from build123d import *

# Parameters (mm, degrees)
BOSS_EXTRUDE1_DEPTH = 5
CUT_EXTRUDE1_REACH  = 58.403
SKETCH2_R           = 1.75
SKETCH4_W           = 75
SKETCH4_H           = 60
BOSS_EXTRUDE2_DEPTH = 5
CUT_EXTRUDE2_REACH  = 90.459
SKETCH3_R           = 2.5
SKETCH3_W           = 23
SKETCH3_H           = 42
FILLET1_R           = 25
FILLET2_R           = 5
FILLET3_R           = 2
FILLET4_R           = 1
BOSS_EXTRUDE3_DEPTH = 10
LPATTERN1_COUNT     = 2
LPATTERN1_PITCH     = 50
CUT_EXTRUDE3_REACH  = 95.708
SKETCH7_R           = 5


with BuildPart() as part:
    # Sketch1 → Boss-Extrude1 (new body)
    with BuildSketch(Plane(origin=(0, 0, 0), x_dir=(0, 0, -1), z_dir=(1, 0, 0))):
        with BuildLine():
            ThreePointArc((-30, -17.5), (0, -47.5), (30, -17.5))
            Line((30, -17.5), (30, 17.5))
            Line((30, 17.5), (-30, 17.5))
            Line((-30, 17.5), (-30, -17.5))
        make_face()
    extrude(amount=BOSS_EXTRUDE1_DEPTH)

    # Sketch2 → Cut-Extrude1 (cut, up to next)
    with BuildSketch(Plane(origin=(5, 0, 0), x_dir=(0, 0, -1), z_dir=(1, 0, 0)), mode=Mode.PRIVATE) as cut_extrude1_sk1:
        with Locations((-15, -32.5)):
            Circle(SKETCH2_R)
    cut_extrude1_tool1 = extrude(cut_extrude1_sk1.sketch, amount=-CUT_EXTRUDE1_REACH, mode=Mode.PRIVATE) & part.part
    # Sketch2 → Cut-Extrude1 (cut, up to next)
    with BuildSketch(Plane(origin=(5, 0, 0), x_dir=(0, 0, -1), z_dir=(1, 0, 0)), mode=Mode.PRIVATE) as cut_extrude1_sk2:
        with Locations((15, -32.5)):
            Circle(SKETCH2_R)
    cut_extrude1_tool2 = extrude(cut_extrude1_sk2.sketch, amount=-CUT_EXTRUDE1_REACH, mode=Mode.PRIVATE) & part.part
    # Sketch2 → Cut-Extrude1 (cut, up to next)
    with BuildSketch(Plane(origin=(5, 0, 0), x_dir=(0, 0, -1), z_dir=(1, 0, 0)), mode=Mode.PRIVATE) as cut_extrude1_sk3:
        with Locations((-15, -2.5)):
            Circle(SKETCH2_R)
    cut_extrude1_tool3 = extrude(cut_extrude1_sk3.sketch, amount=-CUT_EXTRUDE1_REACH, mode=Mode.PRIVATE) & part.part
    # Sketch2 → Cut-Extrude1 (cut, up to next)
    with BuildSketch(Plane(origin=(5, 0, 0), x_dir=(0, 0, -1), z_dir=(1, 0, 0)), mode=Mode.PRIVATE) as cut_extrude1_sk4:
        with Locations((0, -2.5)):
            Circle(SKETCH2_R)
    cut_extrude1_tool4 = extrude(cut_extrude1_sk4.sketch, amount=-CUT_EXTRUDE1_REACH, mode=Mode.PRIVATE) & part.part
    # Sketch2 → Cut-Extrude1 (cut, up to next)
    with BuildSketch(Plane(origin=(5, 0, 0), x_dir=(0, 0, -1), z_dir=(1, 0, 0)), mode=Mode.PRIVATE) as cut_extrude1_sk5:
        with Locations((15, -2.5)):
            Circle(SKETCH2_R)
    cut_extrude1_tool5 = extrude(cut_extrude1_sk5.sketch, amount=-CUT_EXTRUDE1_REACH, mode=Mode.PRIVATE) & part.part
    # Sketch2 → Cut-Extrude1 (cut, up to next)
    with BuildSketch(Plane(origin=(5, 0, 0), x_dir=(0, 0, -1), z_dir=(1, 0, 0)), mode=Mode.PRIVATE) as cut_extrude1_sk6:
        with Locations((0, -32.5)):
            Circle(SKETCH2_R)
    cut_extrude1_tool6 = extrude(cut_extrude1_sk6.sketch, amount=-CUT_EXTRUDE1_REACH, mode=Mode.PRIVATE) & part.part
    # Sketch2 → Cut-Extrude1 (cut, up to next)
    with BuildSketch(Plane(origin=(5, 0, 0), x_dir=(0, 0, -1), z_dir=(1, 0, 0)), mode=Mode.PRIVATE) as cut_extrude1_sk7:
        with Locations((-15, -17.5)):
            Circle(SKETCH2_R)
    cut_extrude1_tool7 = extrude(cut_extrude1_sk7.sketch, amount=-CUT_EXTRUDE1_REACH, mode=Mode.PRIVATE) & part.part
    # Sketch2 → Cut-Extrude1 (cut, up to next)
    with BuildSketch(Plane(origin=(5, 0, 0), x_dir=(0, 0, -1), z_dir=(1, 0, 0)), mode=Mode.PRIVATE) as cut_extrude1_sk8:
        with Locations((15, -17.5)):
            Circle(SKETCH2_R)
    cut_extrude1_tool8 = extrude(cut_extrude1_sk8.sketch, amount=-CUT_EXTRUDE1_REACH, mode=Mode.PRIVATE) & part.part
    add(cut_extrude1_tool1.solids().sort_by_distance((5, -32.5, 15))[0], mode=Mode.SUBTRACT)
    add(cut_extrude1_tool2.solids().sort_by_distance((5, -32.5, -15))[0], mode=Mode.SUBTRACT)
    add(cut_extrude1_tool3.solids().sort_by_distance((5, -2.5, 15))[0], mode=Mode.SUBTRACT)
    add(cut_extrude1_tool4.solids().sort_by_distance((5, -2.5, 0))[0], mode=Mode.SUBTRACT)
    add(cut_extrude1_tool5.solids().sort_by_distance((5, -2.5, -15))[0], mode=Mode.SUBTRACT)
    add(cut_extrude1_tool6.solids().sort_by_distance((5, -32.5, 0))[0], mode=Mode.SUBTRACT)
    add(cut_extrude1_tool7.solids().sort_by_distance((5, -17.5, 15))[0], mode=Mode.SUBTRACT)
    add(cut_extrude1_tool8.solids().sort_by_distance((5, -17.5, -15))[0], mode=Mode.SUBTRACT)

    # Sketch4 → Boss-Extrude2 (add)
    with BuildSketch(Plane(origin=(0, 17.5, 0), x_dir=(1, 0, 0), z_dir=(0, 1, 0))):
        with Locations((37.5, 0)):
            Rectangle(SKETCH4_W, SKETCH4_H)
    extrude(amount=BOSS_EXTRUDE2_DEPTH)

    # Sketch3 → Cut-Extrude2 (cut, up to next)
    with BuildSketch(Plane(origin=(30, 22.5, 0), x_dir=(0, 0, -1), z_dir=(0, 1, 0)), mode=Mode.PRIVATE) as cut_extrude2_sk1:
        with Locations(Location((-5.25, 17.65, 0), (0, 0, 180))):
            Circle(SKETCH3_R)
    cut_extrude2_tool1 = extrude(cut_extrude2_sk1.sketch, amount=-CUT_EXTRUDE2_REACH, mode=Mode.PRIVATE) & part.part
    # Sketch3 → Cut-Extrude2 (cut, up to next)
    with BuildSketch(Plane(origin=(30, 22.5, 0), x_dir=(0, 0, -1), z_dir=(0, 1, 0)), mode=Mode.PRIVATE) as cut_extrude2_sk2:
        with Locations(Location((5.25, 17.65, 0), (0, 0, 180))):
            Circle(SKETCH3_R)
    cut_extrude2_tool2 = extrude(cut_extrude2_sk2.sketch, amount=-CUT_EXTRUDE2_REACH, mode=Mode.PRIVATE) & part.part
    # Sketch3 → Cut-Extrude2 (cut, up to next)
    with BuildSketch(Plane(origin=(30, 22.5, 0), x_dir=(0, 0, -1), z_dir=(0, 1, 0)), mode=Mode.PRIVATE) as cut_extrude2_sk3:
        with Locations(Location((5.25, -32.65, 0), (0, 0, 180))):
            Circle(SKETCH3_R)
    cut_extrude2_tool3 = extrude(cut_extrude2_sk3.sketch, amount=-CUT_EXTRUDE2_REACH, mode=Mode.PRIVATE) & part.part
    # Sketch3 → Cut-Extrude2 (cut, up to next)
    with BuildSketch(Plane(origin=(30, 22.5, 0), x_dir=(0, 0, -1), z_dir=(0, 1, 0)), mode=Mode.PRIVATE) as cut_extrude2_sk4:
        with Locations(Location((-5.25, -32.65, 0), (0, 0, 180))):
            Circle(SKETCH3_R)
    cut_extrude2_tool4 = extrude(cut_extrude2_sk4.sketch, amount=-CUT_EXTRUDE2_REACH, mode=Mode.PRIVATE) & part.part
    # Sketch3 → Cut-Extrude2 (cut, up to next)
    with BuildSketch(Plane(origin=(30, 22.5, 0), x_dir=(0, 0, -1), z_dir=(0, 1, 0)), mode=Mode.PRIVATE) as cut_extrude2_sk5:
        with Locations((0, -7.5)):
            Rectangle(SKETCH3_W, SKETCH3_H)
    cut_extrude2_tool5 = extrude(cut_extrude2_sk5.sketch, amount=-CUT_EXTRUDE2_REACH, mode=Mode.PRIVATE) & part.part
    add(cut_extrude2_tool1.solids().sort_by_distance((12.35, 22.5, 5.25))[0], mode=Mode.SUBTRACT)
    add(cut_extrude2_tool2.solids().sort_by_distance((12.35, 22.5, -5.25))[0], mode=Mode.SUBTRACT)
    add(cut_extrude2_tool3.solids().sort_by_distance((62.65, 22.5, -5.25))[0], mode=Mode.SUBTRACT)
    add(cut_extrude2_tool4.solids().sort_by_distance((62.65, 22.5, 5.25))[0], mode=Mode.SUBTRACT)
    add(cut_extrude2_tool5.solids().sort_by_distance((37.5, 22.5, 0))[0], mode=Mode.SUBTRACT)

    # Fillet1
    fillet1_edges = [part.edges().sort_by_distance(p)[0] for p in [
        (75, 20, 30),
        (75, 20, -30),
    ]]
    fillet(fillet1_edges, radius=FILLET1_R)

    # Fillet2
    fillet2_edges = [part.edges().sort_by_distance(p)[0] for p in [
        (0, 22.5, 0),
    ]]
    fillet(fillet2_edges, radius=FILLET2_R)

    # Fillet3
    fillet3_edges = [part.edges().sort_by_distance(p)[0] for p in [
        (5, 17.5, 0),
    ]]
    fillet(fillet3_edges, radius=FILLET3_R)

    # Fillet4
    fillet4_edges = [part.edges().sort_by_distance(p)[0] for p in [
        (58.5, 20, -11.5),
        (58.5, 20, 11.5),
        (16.5, 20, 11.5),
        (16.5, 20, -11.5),
    ]]
    fillet(fillet4_edges, radius=FILLET4_R)

    # Sketch6 → Boss-Extrude3 (add)
    with BuildSketch(Plane.XY.offset(30)):
        Polygon((18.5, 17.5), (5, 2.743645437), (5, 17.5), align=None)
    boss_extrude3 = extrude(amount=-BOSS_EXTRUDE3_DEPTH)

    # LPattern1: Boss-Extrude3 ×2
    with Locations(*[(0, 0, -i * LPATTERN1_PITCH) for i in range(1, LPATTERN1_COUNT)]):
        add(boss_extrude3)

    # Sketch7 → Cut-Extrude3 (cut, up to next)
    with BuildSketch(Plane.ZY, mode=Mode.PRIVATE) as cut_extrude3_sk1:
        with Locations((0, -17.5)):
            Circle(SKETCH7_R)
    cut_extrude3_tool1 = extrude(cut_extrude3_sk1.sketch, amount=-CUT_EXTRUDE3_REACH, mode=Mode.PRIVATE) & part.part
    add(cut_extrude3_tool1.solids().sort_by_distance((0, -17.5, 0))[0], mode=Mode.SUBTRACT)


solid = part.part
Part model, mm, in its own coordinate system. A direction names the side the tool comes from. Coordinates: 2 decimals unless noted, no trailing zeros. Loops run counter-clockwise (first coordinate to the right, second up) from the corner with the lowest first, then second, coordinate; pieces in that order, holes last. Notation, with made-up numbers: (-22.5, 84) - (32.5, 84) arc R24 ccw to (32.5, 113) - close; hole circle Ø5 at (49.25, 16). An arc over 180 degrees is marked (long way). Write each question's results on one line, items separated by ' | '. Start each with the question number.
Q1. Drop flat-ended pins along their axis: pin 1 Ø2 at (y, z) = (-17.5, 15) entering from -X; pin 2 Ø8 at (x, z) = (23.5, -24) entering from -Y; pin 3 Ø6 at (y, z) = (-8.5, -13) entering from +X. Give the stop position or say it passes through.
Q2. Slice it at A-A on x = 34.5. Give the cut face in (y, z).
Q3. Slice it at B-B on z = 0. Give the cut face in (x, y).
Q4. Probe line 1 along Z through (x, y) = (2, -32); line 2 along X through (y, z) = (19.1, 5.25); line 3 along Y through (x, z) = (2, -15). List the from-to ranges inside material, lowest first.
Q5. Slice it at D-D on z = -15. Give the cut face in (x, y), and give its area (3 significant figures).
Q6. Slice it at C-C on y = -32.5. Give the cut face in (x, z), and give its area (3 significant figures).
Q7. Which spindle directions (+Z, -Z, +X, -X, +Y, -Y) get a long thin tool onto all of the face, cutting with end or side? Do faces 4 (the flat face through (38, 20, -11.5)), 5 (the cylindrical face through (2.54, -4.21, 0.38)), 6 (the flat face through (41, 17.5, 13)). Say none if no direction does.
Q8. Two-plate mould, pull along Z, no slides. Class faces 1 (the flat face through (14, 13, 30)), 2 (the cylindrical face through (60.21, 20.04, -5.79)), 3 (the cylindrical face through (1.5, 21.07, -0.42)): +Z half, -Z half, draft (parallel to the pull), parting line (faces both ways), or undercut.
Answer:
1) pin 1: passes through | pin 2: stops at y = 17.5 | pin 3: stops at x = 5
2) outline: (17.5, -30) - (22.5, -30) - (22.5, -11.5) - (17.5, -11.5) - close; (17.5, 11.5) - (22.5, 11.5) - (22.5, 30) - (17.5, 30) - close
3) outline: (0, -47.5) - (5, -47.5) - (5, -34.25) - (0, -34.25) - close; (0, -30.75) - (5, -30.75) - (5, -22.5) - (0, -22.5) - close; (0, -12.5) - (5, -12.5) - (5, -4.25) - (0, -4.25) - close; (0, -0.75) - (5, -0.75) - (5, 15.5) arc R2 cw to (7, 17.5) - (16.5, 17.5) - (16.5, 22.5) - (5, 22.5) arc R5 ccw to (0, 17.5) - close; (58.5, 17.5) - (75, 17.5) - (75, 22.5) - (58.5, 22.5) - close
4) line 1: z = -26.26 to -16.68, -13.32 to -1.68, 1.68 to 13.32, 16.68 to 26.26 | line 2: x = 0.26 to 9.85, 14.85 to 16.5, 58.5 to 60.15, 65.15 to 75 | line 3: y = -43.48 to -34.25, -30.75 to -19.25, -15.75 to -4.25, -0.75 to 21.5
5) outline: (0, -43.48) - (5, -43.48) - (5, -34.25) - (0, -34.25) - close; (0, -30.75) - (5, -30.75) - (5, -19.25) - (0, -19.25) - close; (0, -15.75) - (5, -15.75) - (5, -4.25) - (0, -4.25) - close; (0, -0.75) - (5, -0.75) - (5, 15.5) arc R2 cw to (7, 17.5) - (72.91, 17.5) - (72.91, 22.5) - (5, 22.5) arc R5 ccw to (0, 17.5) - close | area: 612 mm2
6) outline: (0, -25.98) - (5, -25.98) - (5, -16.75) - (0, -16.75) - close; (0, -13.25) - (5, -13.25) - (5, -1.75) - (0, -1.75) - close; (0, 1.75) - (5, 1.75) - (5, 13.25) - (0, 13.25) - close; (0, 16.75) - (5, 16.75) - (5, 25.98) - (0, 25.98) - close | area: 207 mm2
7) face 4: +Y, -Y | face 5: +X, -X | face 6: +X, -Y
8) face 1: +Z half | face 2: undercut | face 3: draft
